Could you check a few things on this model? Use its own coordinates, in mm. Face numbers are marked on the shaded views. A direction names the side the tool comes from. Give positions to 0.01 mm unless a question says otherwise; leave off trailing zeros. Loops run counter-clockwise (first coordinate to the right, second up) from the corner with the lowest first, then second, coordinate; pieces in that order, holes last. Notation, with made-up numbers: M -28.75,65.25 L -24.75,65.25 A23 ccw -24.75,96.25 Z; hole C 26,16.5 d2. An arc over 180 degrees is marked long. Answer in a Markdown table with one row per item. Add a question column.
1. If we section it at B-B on z = 21.3: List the corners of the cut face in (x, y) for me, then the cut area to 4 significant figures.
2. If we section it at D-D on y = -10: List the corners of the cut face in (x, z) for me, then the cut area to 3 significant figures.
3. If we section it at A-A on z = 5.8: List the corners of the cut face in (x, y) for me, then the cut area to 4 significant figures.
4. Which directions (+Z, -Z, +X, -X, +Y, -Y) give clear straight access to the entire face, cutting with the end or side of a thin tool? Please do the marked faces 1, 2, 3, 4 and 5.
5. If we section it at C-C on x = 17.5: List the corners of the cut face in (y, z) for me, then the cut area to 3 significant figures.
6. I need wall thicknesses on line 1 along X through (y, z) = (1.3, 5.8); line 2 along Z through (x, y) = (36.8, -1.2); line 3 along X through (y, z) = (16, 22). Which ranges of each line are inside material? Lowest first, please. Write a range as from..to.
7. I'm going to push flat-ended pins straight in: pin 1 Ø14 at (x, y) = (15, -10) entering from +Z; pin 2 Ø3 at (x, z) = (37.5, 28.5) entering from +Y; pin 3 Ø4.5 at (x, z) = (5.8, 36.8) entering from -Y. Where does each tip first touch, or does it pass through?
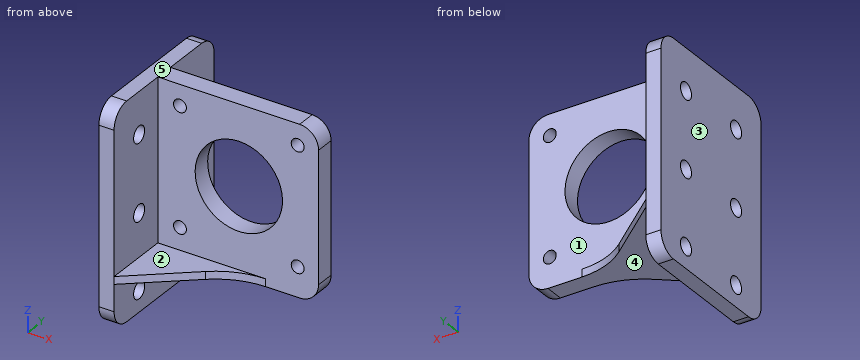
```python
from build123d import *

# Parameters (mm, degrees)
SKETCH_1_W                      = 42.3
SKETCH_1_H                      = 5
SKETCH_1_W_2                    = 21.15
EXTRUDE_1_DEPTH                 = 42.3
CUT_EXTRUDE_1_REACH             = 65.076
SKETCH_2_R                      = 11.5
SKETCH_2_R_2                    = 1.7
CUT_EXTRUDE_1_DIRECTION_2_REACH = 65.076
SKETCH_1_3_W                    = 42.3
SKETCH_1_3_H                    = 5
SKETCH_1_3_W_2                  = 21.15
EXTRUDE_2_DEPTH                 = 2
EXTRUDE_START                   = -2
EXTRUDE_3_DEPTH                 = 12
CUT_EXTRUDE_2_REACH             = 65.076
SKETCH_4_R                      = 2.2
FILLET_1_R                      = 5
FILLET_2_R                      = 20


with BuildPart() as part:
    # 草图1 → 凸台-拉伸1 (new body)
    with BuildSketch(Plane.XY):
        Polygon((0, 2.5), (0, -2.5), (0, -20), (-4, -20), (-4, 20), (0, 20), align=None)
        with Locations((21.15, 0)):
            Rectangle(SKETCH_1_W, SKETCH_1_H)
        Polygon((-4, 0), (0, 0), (0, 2.5), (0, 20), (-4, 20), align=None)
        with Locations((31.725, 0)):
            Rectangle(SKETCH_1_W_2, SKETCH_1_H)
    extrude(amount=EXTRUDE_1_DEPTH)

    # 草图2 → 切除-拉伸1 (cut, up to next)
    with BuildSketch(Plane(origin=(0, 0, 0), x_dir=(1, 0, 0), z_dir=(0, 1, 0)), mode=Mode.PRIVATE) as cut_extrude_1_sk1:
        with Locations(Location((21.3, -21.3, 0), (0, 0, 270))):
            Circle(SKETCH_2_R)
    cut_extrude_1_tool1 = extrude(cut_extrude_1_sk1.sketch, amount=CUT_EXTRUDE_1_REACH, mode=Mode.PRIVATE) & part.part
    # 草图2 → 切除-拉伸1 (cut, up to next)
    with BuildSketch(Plane(origin=(0, 0, 0), x_dir=(1, 0, 0), z_dir=(0, 1, 0)), mode=Mode.PRIVATE) as cut_extrude_1_sk2:
        with Locations(Location((36.8, -5.8, 0), (0, 0, 270))):
            Circle(SKETCH_2_R_2)
    cut_extrude_1_tool2 = extrude(cut_extrude_1_sk2.sketch, amount=CUT_EXTRUDE_1_REACH, mode=Mode.PRIVATE) & part.part
    # 草图2 → 切除-拉伸1 (cut, up to next)
    with BuildSketch(Plane(origin=(0, 0, 0), x_dir=(1, 0, 0), z_dir=(0, 1, 0)), mode=Mode.PRIVATE) as cut_extrude_1_sk3:
        with Locations(Location((36.8, -36.8, 0), (0, 0, 270))):
            Circle(SKETCH_2_R_2)
    cut_extrude_1_tool3 = extrude(cut_extrude_1_sk3.sketch, amount=CUT_EXTRUDE_1_REACH, mode=Mode.PRIVATE) & part.part
    # 草图2 → 切除-拉伸1 (cut, up to next)
    with BuildSketch(Plane(origin=(0, 0, 0), x_dir=(1, 0, 0), z_dir=(0, 1, 0)), mode=Mode.PRIVATE) as cut_extrude_1_sk4:
        with Locations(Location((5.8, -36.8, 0), (0, 0, 270))):
            Circle(SKETCH_2_R_2)
    cut_extrude_1_tool4 = extrude(cut_extrude_1_sk4.sketch, amount=CUT_EXTRUDE_1_REACH, mode=Mode.PRIVATE) & part.part
    # 草图2 → 切除-拉伸1 (cut, up to next)
    with BuildSketch(Plane(origin=(0, 0, 0), x_dir=(1, 0, 0), z_dir=(0, 1, 0)), mode=Mode.PRIVATE) as cut_extrude_1_sk5:
        with Locations(Location((5.8, -5.8, 0), (0, 0, 270))):
            Circle(SKETCH_2_R_2)
    cut_extrude_1_tool5 = extrude(cut_extrude_1_sk5.sketch, amount=CUT_EXTRUDE_1_REACH, mode=Mode.PRIVATE) & part.part
    add(cut_extrude_1_tool1.solids().sort_by_distance((21.3, 0, 21.3))[0], mode=Mode.SUBTRACT)
    add(cut_extrude_1_tool2.solids().sort_by_distance((36.8, 0, 5.8))[0], mode=Mode.SUBTRACT)
    add(cut_extrude_1_tool3.solids().sort_by_distance((36.8, 0, 36.8))[0], mode=Mode.SUBTRACT)
    add(cut_extrude_1_tool4.solids().sort_by_distance((5.8, 0, 36.8))[0], mode=Mode.SUBTRACT)
    add(cut_extrude_1_tool5.solids().sort_by_distance((5.8, 0, 5.8))[0], mode=Mode.SUBTRACT)

    # 草图2 → 切除-拉伸1 direction 2 (cut, up to next)
    with BuildSketch(Plane(origin=(0, 0, 0), x_dir=(1, 0, 0), z_dir=(0, 1, 0)), mode=Mode.PRIVATE) as cut_extrude_1_direction_2_sk1:
        with Locations(Location((21.3, -21.3, 0), (0, 0, 270))):
            Circle(SKETCH_2_R)
    cut_extrude_1_direction_2_tool1 = extrude(cut_extrude_1_direction_2_sk1.sketch, amount=-CUT_EXTRUDE_1_DIRECTION_2_REACH, mode=Mode.PRIVATE) & part.part
    # 草图2 → 切除-拉伸1 direction 2 (cut, up to next)
    with BuildSketch(Plane(origin=(0, 0, 0), x_dir=(1, 0, 0), z_dir=(0, 1, 0)), mode=Mode.PRIVATE) as cut_extrude_1_direction_2_sk2:
        with Locations(Location((36.8, -5.8, 0), (0, 0, 270))):
            Circle(SKETCH_2_R_2)
    cut_extrude_1_direction_2_tool2 = extrude(cut_extrude_1_direction_2_sk2.sketch, amount=-CUT_EXTRUDE_1_DIRECTION_2_REACH, mode=Mode.PRIVATE) & part.part
    # 草图2 → 切除-拉伸1 direction 2 (cut, up to next)
    with BuildSketch(Plane(origin=(0, 0, 0), x_dir=(1, 0, 0), z_dir=(0, 1, 0)), mode=Mode.PRIVATE) as cut_extrude_1_direction_2_sk3:
        with Locations(Location((36.8, -36.8, 0), (0, 0, 270))):
            Circle(SKETCH_2_R_2)
    cut_extrude_1_direction_2_tool3 = extrude(cut_extrude_1_direction_2_sk3.sketch, amount=-CUT_EXTRUDE_1_DIRECTION_2_REACH, mode=Mode.PRIVATE) & part.part
    # 草图2 → 切除-拉伸1 direction 2 (cut, up to next)
    with BuildSketch(Plane(origin=(0, 0, 0), x_dir=(1, 0, 0), z_dir=(0, 1, 0)), mode=Mode.PRIVATE) as cut_extrude_1_direction_2_sk4:
        with Locations(Location((5.8, -36.8, 0), (0, 0, 270))):
            Circle(SKETCH_2_R_2)
    cut_extrude_1_direction_2_tool4 = extrude(cut_extrude_1_direction_2_sk4.sketch, amount=-CUT_EXTRUDE_1_DIRECTION_2_REACH, mode=Mode.PRIVATE) & part.part
    # 草图2 → 切除-拉伸1 direction 2 (cut, up to next)
    with BuildSketch(Plane(origin=(0, 0, 0), x_dir=(1, 0, 0), z_dir=(0, 1, 0)), mode=Mode.PRIVATE) as cut_extrude_1_direction_2_sk5:
        with Locations(Location((5.8, -5.8, 0), (0, 0, 270))):
            Circle(SKETCH_2_R_2)
    cut_extrude_1_direction_2_tool5 = extrude(cut_extrude_1_direction_2_sk5.sketch, amount=-CUT_EXTRUDE_1_DIRECTION_2_REACH, mode=Mode.PRIVATE) & part.part
    add(cut_extrude_1_direction_2_tool1.solids().sort_by_distance((21.3, 0, 21.3))[0], mode=Mode.SUBTRACT)
    add(cut_extrude_1_direction_2_tool2.solids().sort_by_distance((36.8, 0, 5.8))[0], mode=Mode.SUBTRACT)
    add(cut_extrude_1_direction_2_tool3.solids().sort_by_distance((36.8, 0, 36.8))[0], mode=Mode.SUBTRACT)
    add(cut_extrude_1_direction_2_tool4.solids().sort_by_distance((5.8, 0, 36.8))[0], mode=Mode.SUBTRACT)
    add(cut_extrude_1_direction_2_tool5.solids().sort_by_distance((5.8, 0, 5.8))[0], mode=Mode.SUBTRACT)

    # 草图1<3> → 凸台-拉伸2 (add)
    with BuildSketch(Plane.XY):
        Polygon((0, 2.5), (21.15, 2.5), (0, 20), align=None)
        Polygon((21.15, -2.5), (0, -2.5), (0, -20), align=None)
        Polygon((0, -20), (0, -2.5), (0, 0), (-4, 0), (-4, -20), align=None)
        Polygon((-4, 0), (0, 0), (0, 2.5), (0, 20), (-4, 20), align=None)
        with Locations((21.15, 0)):
            Rectangle(SKETCH_1_3_W, SKETCH_1_3_H)
        with Locations((31.725, 0)):
            Rectangle(SKETCH_1_3_W_2, SKETCH_1_3_H)
    extrude(amount=-EXTRUDE_2_DEPTH)

    # 草图1<4> → 凸台-拉伸3 (add)
    with BuildSketch(Plane.XY.offset(EXTRUDE_START)):
        Polygon((-4, 0), (0, 0), (0, 2.5), (0, 20), (-4, 20), align=None)
        Polygon((0, -20), (0, -2.5), (0, 0), (-4, 0), (-4, -20), align=None)
    extrude(amount=-EXTRUDE_3_DEPTH)

    # 草图4 → 切除-拉伸2 (cut, up to next)
    with BuildSketch(Plane(origin=(0, 0, 0), x_dir=(0, 0, -1), z_dir=(1, 0, 0)), mode=Mode.PRIVATE) as cut_extrude_2_sk1:
        with Locations((8.4, 10)):
            Circle(SKETCH_4_R)
    cut_extrude_2_tool1 = extrude(cut_extrude_2_sk1.sketch, amount=-CUT_EXTRUDE_2_REACH, mode=Mode.PRIVATE) & part.part
    # 草图4 → 切除-拉伸2 (cut, up to next)
    with BuildSketch(Plane(origin=(0, 0, 0), x_dir=(0, 0, -1), z_dir=(1, 0, 0)), mode=Mode.PRIVATE) as cut_extrude_2_sk2:
        with Locations(Location((8.4, -10, 0), (0, 0, 90))):
            Circle(SKETCH_4_R)
    cut_extrude_2_tool2 = extrude(cut_extrude_2_sk2.sketch, amount=-CUT_EXTRUDE_2_REACH, mode=Mode.PRIVATE) & part.part
    # 草图4 → 切除-拉伸2 (cut, up to next)
    with BuildSketch(Plane(origin=(0, 0, 0), x_dir=(0, 0, -1), z_dir=(1, 0, 0)), mode=Mode.PRIVATE) as cut_extrude_2_sk3:
        with Locations(Location((-11.3, 10, 0), (0, 0, 90))):
            Circle(SKETCH_4_R)
    cut_extrude_2_tool3 = extrude(cut_extrude_2_sk3.sketch, amount=-CUT_EXTRUDE_2_REACH, mode=Mode.PRIVATE) & part.part
    # 草图4 → 切除-拉伸2 (cut, up to next)
    with BuildSketch(Plane(origin=(0, 0, 0), x_dir=(0, 0, -1), z_dir=(1, 0, 0)), mode=Mode.PRIVATE) as cut_extrude_2_sk4:
        with Locations((-11.3, -10)):
            Circle(SKETCH_4_R)
    cut_extrude_2_tool4 = extrude(cut_extrude_2_sk4.sketch, amount=-CUT_EXTRUDE_2_REACH, mode=Mode.PRIVATE) & part.part
    # 草图4 → 切除-拉伸2 (cut, up to next)
    with BuildSketch(Plane(origin=(0, 0, 0), x_dir=(0, 0, -1), z_dir=(1, 0, 0)), mode=Mode.PRIVATE) as cut_extrude_2_sk5:
        with Locations((-31.3, 10)):
            Circle(SKETCH_4_R)
    cut_extrude_2_tool5 = extrude(cut_extrude_2_sk5.sketch, amount=-CUT_EXTRUDE_2_REACH, mode=Mode.PRIVATE) & part.part
    # 草图4 → 切除-拉伸2 (cut, up to next)
    with BuildSketch(Plane(origin=(0, 0, 0), x_dir=(0, 0, -1), z_dir=(1, 0, 0)), mode=Mode.PRIVATE) as cut_extrude_2_sk6:
        with Locations(Location((-31.3, -10, 0), (0, 0, 90))):
            Circle(SKETCH_4_R)
    cut_extrude_2_tool6 = extrude(cut_extrude_2_sk6.sketch, amount=-CUT_EXTRUDE_2_REACH, mode=Mode.PRIVATE) & part.part
    add(cut_extrude_2_tool1.solids().sort_by_distance((0, 10, -8.4))[0], mode=Mode.SUBTRACT)
    add(cut_extrude_2_tool2.solids().sort_by_distance((0, -10, -8.4))[0], mode=Mode.SUBTRACT)
    add(cut_extrude_2_tool3.solids().sort_by_distance((0, 10, 11.3))[0], mode=Mode.SUBTRACT)
    add(cut_extrude_2_tool4.solids().sort_by_distance((0, -10, 11.3))[0], mode=Mode.SUBTRACT)
    add(cut_extrude_2_tool5.solids().sort_by_distance((0, 10, 31.3))[0], mode=Mode.SUBTRACT)
    add(cut_extrude_2_tool6.solids().sort_by_distance((0, -10, 31.3))[0], mode=Mode.SUBTRACT)

    # 圆角1
    fillet_1_edges = [part.edges().sort_by_distance(p)[0] for p in [
        (42.3, 0, 42.3),
        (-2, 20, 42.3),
        (-2, -20, 42.3),
        (42.3, 0, -2),
        (-2, -20, -14),
        (-2, 20, -14),
    ]]
    fillet(fillet_1_edges, radius=FILLET_1_R)

    # 圆角2
    fillet_2_edges = [part.edges().sort_by_distance(p)[0] for p in [
        (21.15, 2.5, -1),
        (21.15, -2.5, -1),
    ]]
    fillet(fillet_2_edges, radius=FILLET_2_R)


solid = part.part
```
Results:
| question | item | result |
|---|---|---|
| 1 | outline | M -4,-20 L 0,-20 L 0,-2.5 L 9.8,-2.5 L 9.8,2.5 L 0,2.5 L 0,20 L -4,20 Z; M 32.8,-2.5 L 42.3,-2.5 L 42.3,2.5 L 32.8,2.5 Z |
| 1 | area | 256.5 mm2 |
| 2 | outline | M -4,-14 L 0,-14 L 0,-10.6 L -4,-10.6 Z; M -4,-6.2 L 0,-6.2 L 0,-2 L 12.09,-2 L 12.09,0 L 0,0 L 0,9.1 L -4,9.1 Z; M -4,13.5 L 0,13.5 L 0,29.1 L -4,29.1 Z; M -4,33.5 L 0,33.5 L 0,42.3 L -4,42.3 Z |
| 2 | area | 197 mm2 |
| 3 | outline | M -4,-20 L 0,-20 L 0,-2.5 L 4.1,-2.5 L 4.1,2.5 L 0,2.5 L 0,20 L -4,20 Z; M 7.5,-2.5 L 35.1,-2.5 L 35.1,2.5 L 7.5,2.5 Z; M 38.5,-2.5 L 42.3,-2.5 L 42.3,2.5 L 38.5,2.5 Z |
| 3 | area | 337.5 mm2 |
| 4 | face 1 | +Z, +X, +Y |
| 4 | face 2 | +Z, +X, -Y |
| 4 | face 3 | +Z, -Z, -X, +Y, -Y |
| 4 | face 4 | -Z, +X, +Y, -Y |
| 4 | face 5 | +Z, +X, -X, +Y, -Y |
| 5 | outline | M -5.7,-2 L 5.7,-2 L 5.7,0 L 2.5,0 L 2.5,10.45 L -2.5,10.45 L -2.5,0 L -5.7,0 Z; M -2.5,32.15 L 2.5,32.15 L 2.5,42.3 L -2.5,42.3 Z |
| 5 | area | 126 mm2 |
| 6 | line 1 | -4..4.1, 7.5..35.1, 38.5..42.3 |
| 6 | line 2 | -2..4.1, 7.5..35.1, 38.5..42.3 |
| 6 | line 3 | -4..0 |
| 7 | pin 1 | z = 0 |
| 7 | pin 2 | y = 2.5 |
| 7 | pin 3 | y = -2.5 |
